Model file for the job. Use its own axes, mm. Face numbers are marked on the shaded views. A direction names the side the tool comes from. Coordinates: 2 decimals unless noted, no trailing zeros. Order: outer loops, then holes, each group sorted by start corner. A loop starts at its lowest first (then second) coordinate and runs counter-clockwise, first axis right, second up. Notation, with made-up numbers: (8.5, 75) -> (54.5, 75) arc R30 cw to (54.5, 97) -> close; hole circle Ø7 at (52.25, 72.5). An arc over 180 degrees is marked (long way). Use CSV: the item, a comma, the result in double quotes. Start each with the question number.
(1) Cut at A-A on y = -52. Write the cut outline in (x, z), plus the area to 3 significant figures.
(2) Cut at C-C on z = 139. Write the cut outline in (x, y).
(3) Pull direction Y, two halves, no side cores. Call the marked faces 4, 5 and 6: pulls with the +Y half, pulls with the -Y half, needs draft (parallel to the pull), parting line crosses it, or undercut.
(4) Probe L1, parallel to X at y = 9, z = 123; L2, parallel to X at y = -4.7, z = 141.65; L3, parallel to Z at x = 15.5, y = -51.85. List the from-to ranges inside material, lowest first.
(5) Pin check, flat tips, straight feed: pin 1 Ø5 at (x, z) = (-14, 124) entering from +Y; pin 2 Ø14.5 at (x, z) = (0, 141.65) entering from +Y; pin 3 Ø3.5 at (x, y) = (14.5, 9.5) entering from +Z; pin 4 Ø1.8 at (x, z) = (15.5, 123.5) entering from +Y. Stop position of each tip, or through.
(6) Cut at D-D on x = 8.5. Write the cut outline in (y, z).
(7) Cut at B-B on x = 0. Write the cut outline in (y, z), plus the area to 3 significant figures.
(8) Tool access for the marked faces 1, 2 and 3: list every direction of +Z, -Z, +X, -X, +Y, -Y with a clear straight run to the whole face (end or side of a thin tool).
```python
from build123d import *

# Parameters (mm, degrees)
SKETCH11_R          = 1.55
SKETCH11_R_2        = 4.5
BOSS_EXTRUDE1_DEPTH = 7
BOSS_EXTRUDE2_DEPTH = 3
SKETCH13_R          = 3.5
CUT_EXTRUDE1_DEPTH  = 3
SKETCH14_R          = 1.55
BOSS_EXTRUDE3_DEPTH = 3
BOSS_EXTRUDE4_START = -3
SKETCH15_R          = 1.55
BOSS_EXTRUDE4_DEPTH = 3


with BuildPart() as part:
    # Sketch11 → Boss-Extrude1 (new body)
    with BuildSketch(Plane(origin=(0, 0, 51.65), x_dir=(1, 0, 0), z_dir=(0, -1, 0))):
        with BuildLine():
            Line((12.5, 90), (12.5, 71.5))
            Line((12.5, 71.5), (-12.5, 71.5))
            Line((-12.5, 71.5), (-12.5, 90))
            ThreePointArc((-12.5, 90), (0, 102.5), (12.5, 90))
        make_face()
        with Locations(Location((-8.5, 90, 0), (0, 0, 270))):
            Circle(SKETCH11_R, mode=Mode.SUBTRACT)
        with Locations(Location((8.5, 90, 0), (0, 0, 270))):
            Circle(SKETCH11_R, mode=Mode.SUBTRACT)
        with Locations(Location((0, 90, 0), (0, 0, 270))):
            Circle(SKETCH11_R_2, mode=Mode.SUBTRACT)
    extrude(amount=BOSS_EXTRUDE1_DEPTH)

    # Sketch12 → Boss-Extrude2 (add)
    with BuildSketch(Plane(origin=(0, 0, 123.15), x_dir=(-1, 0, 0), z_dir=(0, 0, -1))):
        Polygon((-12.5, 0), (-12.5, 11), (-5, 11), (-5, 16), (5, 16), (5, 11), (12.5, 11), (12.5, 0), (12.5, -7), (12.5, -53), (5, -53), (5, -58), (-5, -58), (-5, -53), (-12.5, -53), (-12.5, -7), align=None)
    extrude(amount=BOSS_EXTRUDE2_DEPTH)

    # Sketch13 → Cut-Extrude1 (cut)
    with BuildSketch(Plane(origin=(0, 0, 0), x_dir=(1, 0, 0), z_dir=(0, 1, 0))):
        with Locations(Location((-8.5, -141.65, 0), (0, 0, 270))):
            Circle(SKETCH13_R)
        with Locations(Location((8.5, -141.65, 0), (0, 0, 270))):
            Circle(SKETCH13_R)
    extrude(amount=-CUT_EXTRUDE1_DEPTH, mode=Mode.SUBTRACT)

    # Sketch14 → Boss-Extrude3 (add)
    with BuildSketch(Plane(origin=(0, 11, 0), x_dir=(1, 0, 0), z_dir=(0, 1, 0))):
        with BuildLine():
            Line((15.5, -120.15), (-15.5, -120.15))
            ThreePointArc((-15.5, -120.15), (-18.5, -123.15), (-15.5, -126.15))
            Line((-15.5, -126.15), (-12.5, -126.15))
            Line((-12.5, -126.15), (-9.5, -123.15))
            Line((-9.5, -123.15), (9.5, -123.15))
            Line((9.5, -123.15), (12.5, -126.15))
            Line((12.5, -126.15), (15.5, -126.15))
            ThreePointArc((15.5, -126.15), (18.5, -123.15), (15.5, -120.15))
        make_face()
        with Locations(Location((-15.5, -123.15, 0), (0, 0, 270))):
            Circle(SKETCH14_R, mode=Mode.SUBTRACT)
        with Locations(Location((15.5, -123.15, 0), (0, 0, 270))):
            Circle(SKETCH14_R, mode=Mode.SUBTRACT)
    extrude(amount=-BOSS_EXTRUDE3_DEPTH)

    # Sketch15 → Boss-Extrude4 (add)
    with BuildSketch(Plane(origin=(0, -53, 0), x_dir=(-1, 0, 0), z_dir=(0, -1, 0)).offset(BOSS_EXTRUDE4_START)):
        with BuildLine():
            Line((15.5, -120.15), (-15.5, -120.15))
            ThreePointArc((-15.5, -120.15), (-18.5, -123.15), (-15.5, -126.15))
            Line((-15.5, -126.15), (-12.5, -126.15))
            Line((-12.5, -126.15), (-9.5, -123.15))
            Line((-9.5, -123.15), (9.5, -123.15))
            Line((9.5, -123.15), (12.5, -126.15))
            Line((12.5, -126.15), (15.5, -126.15))
            ThreePointArc((15.5, -126.15), (18.5, -123.15), (15.5, -120.15))
        make_face()
        with Locations(Location((15.5, -123.15, 0), (0, 0, 270))):
            Circle(SKETCH15_R, mode=Mode.SUBTRACT)
        with Locations(Location((-15.5, -123.15, 0), (0, 0, 270))):
            Circle(SKETCH15_R, mode=Mode.SUBTRACT)
    extrude(amount=BOSS_EXTRUDE4_DEPTH)


solid = part.part
```
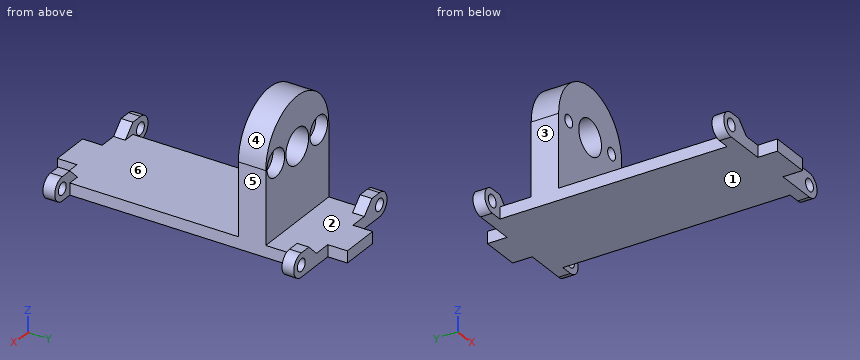
Outcome:
1,outline,"(-15.5, 120.15) -> (15.5, 120.15) arc R3 ccw to (15.5, 126.15) -> (12.5, 126.15) -> (9.5, 123.15) -> (-9.5, 123.15) -> (-12.5, 126.15) -> (-15.5, 126.15) arc R3 ccw to start; hole circle Ø3.1 at (-15.5, 123.15); hole circle Ø3.1 at (15.5, 123.15)"
1,area,"133 mm2"
2,outline,"(-12.5, -7) -> (-3.64, -7) -> (-3.64, 0) -> (-6.21, 0) -> (-6.21, -3) -> (-10.79, -3) -> (-10.79, 0) -> (-12.5, 0) -> close; (3.64, -7) -> (12.5, -7) -> (12.5, 0) -> (10.79, 0) -> (10.79, -3) -> (6.21, -3) -> (6.21, 0) -> (3.64, 0) -> close"
3,face 4,"needs draft"
3,face 5,"undercut"
3,face 6,"undercut"
4,L1,"-18.5 to -17.04, -13.96 to 13.96, 17.04 to 18.5"
4,L2,"-12.5 to -10.05, -6.95 to -4.5, 4.5 to 6.95, 10.05 to 12.5"
4,L3,"120.15 to 121.6, 124.7 to 126.15"
5,pin 1,"y = 11"
5,pin 2,"y = 0"
5,pin 3,"z = 126.15"
5,pin 4,"through"
6,outline,"(-53, 120.15) -> (11, 120.15) -> (11, 123.15) -> (0, 123.15) -> (0, 138.15) -> (-3, 138.15) -> (-3, 140.1) -> (-7, 140.1) -> (-7, 123.15) -> (-53, 123.15) -> close; (-7, 143.2) -> (-3, 143.2) -> (-3, 145.15) -> (0, 145.15) -> (0, 150.82) -> (-7, 150.82) -> close"
7,outline,"(-58, 120.15) -> (16, 120.15) -> (16, 123.15) -> (0, 123.15) -> (0, 137.15) -> (-7, 137.15) -> (-7, 123.15) -> (-58, 123.15) -> close; (-7, 146.15) -> (0, 146.15) -> (0, 154.15) -> (-7, 154.15) -> close"
7,area,"376 mm2"
8,face 1,"-Z, +X, -X, +Y, -Y"
8,face 2,"+Z"
8,face 3,"+Z, -Z, -X"
